Autodesk Inventor part; units mm, degrees
ref_plane "YZ Plane" through (0, 0, 0) normal (1, 0, 0) x (0, 1, 0)
ref_plane "XZ Plane" through (0, 0, 0) normal (0, 1, 0) x (-1, 0, 0)
ref_plane "XY Plane" through (0, 0, 0) normal (0, 0, 1) x (1, 0, 0)
sketch "Sketch1" plane through (0, 0, 0) normal (0, 1, 0) x (-1, 0, 0)
  circle A0 centre (0, 0) radius 1.5
  dimension "d0" = 3
extrude "Extrusion1" add sketch "Sketch1" along normal blind 20
sketch "Sketch2" plane through (0, 20, 0) normal (0, 1, 0) x (1, 0, 0)
  circle A0 centre (0, 0) radius 2.5
  dimension "d3" = 5
extrude "Extrusion2" add sketch "Sketch2" along normal blind 3
fillet "Fillet1" radius 0.2 1 edges at (-2.5, 23, 0)
fillet "Fillet2" radius 0.1 1 edges at (1.5, 0, 0)
properties part number "VIS"
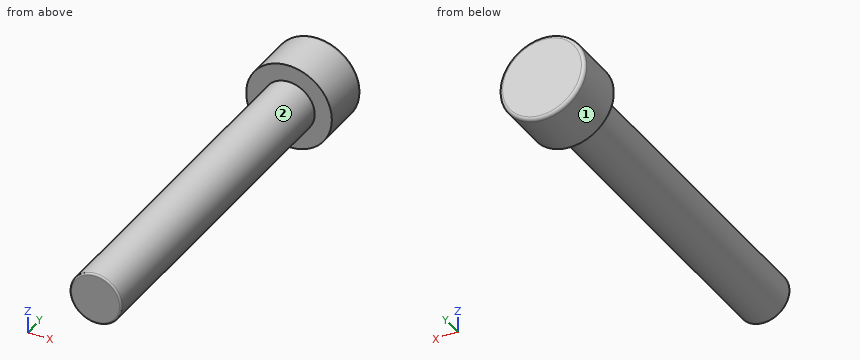
Source: CAD feature listing. Evaluate the final solid. Frame: model axes, mm. Face numbers are marked on the shaded views. A direction names the side the tool comes from. Give positions to 0.01 mm unless a question says otherwise; leave off trailing zeros. Order: outer loops, then holes, each group sorted by start corner. A loop starts at its lowest first (then second) coordinate and runs counter-clockwise, first axis right, second up. Notation, with made-up numbers: (38.5, -21.5) -> (63.5, -21.5) arc R38 ccw to (63.5, 16.5) -> close; hole circle Ø3 at (-30, -34.75). An arc over 180 degrees is marked (long way). Write item = value, one per line.
Item 1: Section query B-B (x = 0). Output: boundary loops of the cut face in (y, z).
Check result:
outline = (0, -1.4) arc R0.1 ccw to (0.1, -1.5) -> (20, -1.5) -> (20, -2.5) -> (22.8, -2.5) arc R0.2 ccw to (23, -2.3) -> (23, 2.3) arc R0.2 ccw to (22.8, 2.5) -> (20, 2.5) -> (20, 1.5) -> (0.1, 1.5) arc R0.1 ccw to (0, 1.4) -> close
Item 2: Ray query, probe 1 along X at (y, z) = (14, 0.1); probe 2 along Y at (x, z) = (2, 1); probe 3 along Z at (x, y) = (0.4, 6.75). Return the intervals inside material, ascending.
Check result:
probe_1 = -1.5 to 1.5
probe_2 = 20 to 23
probe_3 = -1.45 to 1.45
Item 3: Section query A-A (z = 0). Output: boundary loops of the cut face in (x, y).
Check result:
outline = (-2.5, 20) -> (-1.5, 20) -> (-1.5, 0.1) arc R0.1 ccw to (-1.4, 0) -> (1.4, 0) arc R0.1 ccw to (1.5, 0.1) -> (1.5, 20) -> (2.5, 20) -> (2.5, 22.8) arc R0.2 ccw to (2.3, 23) -> (-2.3, 23) arc R0.2 ccw to (-2.5, 22.8) -> close
Item 4: Section query D-D (y = 17.75). Output: boundary loops of the cut face in (x, z).
Check result:
outline = circle Ø3 at (0, 0)
Item 5: Set-up query: the marked faces 1 and 2. Return all of +Z, -Z, +X, -X, +Y, -Y with unobstructed straight access to the full face (end or side cutting, diameter ignored); none if empty.
Check result:
face_1 = +Y, -Y
face_2 = -Y
Item 6: Section query C-C (y = 21.5). Output: boundary loops of the cut face in (x, z).
Check result:
outline = circle Ø5 at (0, 0)
